from build123d import *

# Parameters (mm, degrees)
SKETCH_3_W          = 38
SKETCH_3_H          = 20
EXTRUDE_1_DEPTH     = 6
SKETCH_4_W          = 5
SKETCH_4_H          = 20
EXTRUDE_2_DEPTH     = 59
SKETCH_9_W          = 40.5
SKETCH_9_H          = 24.5
EXTRUDE_4_DEPTH     = 4
SKETCH_12_W         = 21.5
SKETCH_12_H         = 85
EXTRUDE_5_DEPTH     = 4
SKETCH_13_W         = 21.5
SKETCH_13_H         = 51
EXTRUDE_6_DEPTH     = 6
EXTRUDE_8_DEPTH     = 4
CUT_EXTRUDE_START   = -20
CUT_EXTRUDE_7_DEPTH = 8
SKETCH_5_R          = 2.1
CUT_EXTRUDE_1_DEPTH = 114.903467902
CUT_EXTRUDE_2_DEPTH = 3.8
SKETCH_7_R          = 2.6
CUT_EXTRUDE_3_DEPTH = 120.57529009
SKETCH_17_R         = 2.1
CUT_EXTRUDE_4_DEPTH = 165.903001792
CUT_EXTRUDE_5_DEPTH = 3.3
SKETCH_19_R         = 2.5
CUT_EXTRUDE_6_DEPTH = 118.123866056
FILLET_2_R          = 2.5
CHAMFER_2_SIZE      = 4


with BuildPart() as part:
    # Эскиз3 → Бобышка-Вытянуть1 (new body)
    with BuildSketch(Plane.XY):
        Rectangle(SKETCH_3_W, SKETCH_3_H)
    extrude(amount=EXTRUDE_1_DEPTH)

    # Эскиз4 → Бобышка-Вытянуть2 (add)
    with BuildSketch(Plane(origin=(-10.8, 0, 0), x_dir=(1, 0, 0), z_dir=(0, 0, 1))):
        with Locations((10.8, 0)):
            Rectangle(SKETCH_4_W, SKETCH_4_H)
    extrude(amount=-EXTRUDE_2_DEPTH)

    # Эскиз9 → Бобышка-Вытянуть4 (add)
    with BuildSketch(Plane.XY.offset(6)):
        with Locations((-17.75, 22.25)):
            Rectangle(SKETCH_9_W, SKETCH_9_H)
    extrude(amount=-EXTRUDE_4_DEPTH)

    # Эскиз12 → Бобышка-Вытянуть5 (add, symmetric)
    with BuildSketch(Plane(origin=(0, 10, 0), x_dir=(-1, 0, 0), z_dir=(0, 1, 0))):
        with Locations((8.25, 48.5)):
            Rectangle(SKETCH_12_W, SKETCH_12_H)
    extrude(amount=EXTRUDE_5_DEPTH, both=True)

    # Эскиз13 → Бобышка-Вытянуть6 (add)
    with BuildSketch(Plane.XY.offset(91)):
        with Locations((-8.25, 31.5)):
            Rectangle(SKETCH_13_W, SKETCH_13_H)
    extrude(amount=EXTRUDE_6_DEPTH)

    # Эскиз23 → Бобышка-Вытянуть8 (add)
    with BuildSketch(Plane(origin=(0, 10, 0), x_dir=(1, 0, 0), z_dir=(0, 1, 0))):
        Polygon((-2.5, 16.5), (-19, 0), (-2.5, 0), align=None)
    extrude(amount=-EXTRUDE_8_DEPTH)

    # Эскиз21 → Вырез-Вытянуть7 (cut)
    with BuildSketch(Plane(origin=(0, 0, -59), x_dir=(-1, 0, 0), z_dir=(0, 0, -1)).offset(CUT_EXTRUDE_START)):
        with BuildLine():
            Line((1.25, 10), (2.5, 10))
            Line((2.5, 10), (2.5, 8.75))
            ThreePointArc((2.5, 8.75), (2.133883476, 9.633883476), (1.25, 10))
        make_face()
    extrude(amount=-CUT_EXTRUDE_7_DEPTH, mode=Mode.SUBTRACT)

    # Эскиз5 → Вырез-Вытянуть1 (cut, through all)
    with BuildSketch(Plane.XY.offset(6)):
        with Locations((-9, -2)):
            Circle(SKETCH_5_R)
        with Locations((9, -2)):
            Circle(SKETCH_5_R)
    extrude(amount=-CUT_EXTRUDE_1_DEPTH, mode=Mode.SUBTRACT)

    # Эскиз6 → Вырез-Вытянуть2 (cut)
    with BuildSketch(Plane(origin=(0, 0, 0), x_dir=(-1, 0, 0), z_dir=(0, 0, -1))):
        Polygon((-9, 2.156921938), (-12.6, 0.078460969), (-12.6, -4.078460969), (-9, -6.156921938), (-5.4, -4.078460969), (-5.4, 0.078460969), align=None)
        Polygon((9, 2.156921938), (5.4, 0.078460969), (5.4, -4.078460969), (9, -6.156921938), (12.6, -4.078460969), (12.6, 0.078460969), align=None)
    extrude(amount=-CUT_EXTRUDE_2_DEPTH, mode=Mode.SUBTRACT)

    # Эскиз7 → Вырез-Вытянуть3 (cut, through all)
    with BuildSketch(Plane(origin=(2.5, 0, 0), x_dir=(0, 0, -1), z_dir=(1, 0, 0))):
        with Locations(Location((49, 0, 0), (0, 0, 90))):
            Circle(SKETCH_7_R)
    extrude(amount=-CUT_EXTRUDE_3_DEPTH, mode=Mode.SUBTRACT)

    # Эскиз17 → Вырез-Вытянуть4 (cut, through all)
    with BuildSketch(Plane(origin=(0, 0, 91), x_dir=(-1, 0, 0), z_dir=(0, 0, -1))):
        with Locations((7.5, 29)):
            Circle(SKETCH_17_R)
        with Locations((7.5, 47)):
            Circle(SKETCH_17_R)
    extrude(amount=-CUT_EXTRUDE_4_DEPTH, mode=Mode.SUBTRACT)

    # Эскиз18 → Вырез-Вытянуть5 (cut)
    with BuildSketch(Plane.XY.offset(97)):
        Polygon((-3.458548116, 29), (-5.479274058, 32.5), (-9.520725942, 32.5), (-11.541451884, 29), (-9.520725942, 25.5), (-5.479274058, 25.5), align=None)
        Polygon((-3.458548116, 47), (-5.479274058, 50.5), (-9.520725942, 50.5), (-11.541451884, 47), (-9.520725942, 43.5), (-5.479274058, 43.5), align=None)
    extrude(amount=-CUT_EXTRUDE_5_DEPTH, mode=Mode.SUBTRACT)

    # Эскиз19 → Вырез-Вытянуть6 (cut, through all)
    with BuildSketch(Plane(origin=(0, 0, 2), x_dir=(-1, 0, 0), z_dir=(0, 0, -1))):
        with Locations((30.999999999, 27.499999999)):
            Circle(SKETCH_19_R)
    extrude(amount=-CUT_EXTRUDE_6_DEPTH, mode=Mode.SUBTRACT)

    # Скругление2
    fillet_2_edges = [part.edges().sort_by_distance(p)[0] for p in [
        (0, 10, -59),
        (0, -10, -59),
        (2.5, 34.5, 4),
        (-38, 10, 4),
        (-38, 34.5, 4),
        (2.5, 57, 94),
        (-19, 57, 94),
        (19, 10, 3),
        (19, -10, 3),
        (-19, -10, 3),
    ]]
    fillet(fillet_2_edges, radius=FILLET_2_R)

    # Фаска2
    chamfer_2_edges = [part.edges().sort_by_distance(p)[0] for p in [
        (-19, 12, 6),
        (-8.25, 14, 91),
        (-8.25, 14, 6),
    ]]
    chamfer(chamfer_2_edges, length=CHAMFER_2_SIZE)


solid = part.part
Geometry: final body of the model. Coordinates: model frame, mm. A direction names the side the tool comes from. Coordinates: 2 decimals unless noted, no trailing zeros. Order: outer loops, then holes, each group sorted by start corner. A loop starts at its lowest first (then second) coordinate and runs counter-clockwise, first axis right, second up.
1) Section B-B (x = -31). Return loops of the section in (y, z).
Result sheet:
outline: (10, 2) - (25, 2) - (25, 6) - (10, 6) - close; (30, 2) - (34.5, 2) - (34.5, 6) - (30, 6) - close
2) Section D-D (z = 24.5). Return loops of the section in (x, y), then the cut area to 3 significant figures.
Result sheet:
outline: (-19, 6) - (2.5, 6) - (2.5, 14) - (-19, 14) - close
area: 172 mm2
3) Section C-C (x = -15). Return loops of the section in (y, z).
Result sheet:
outline: (-10, 0) - (6, 0) - (6, -4) - (10, -4) - (10, 2) - (34.5, 2) - (34.5, 6) - (18, 6) - (14, 10) - (14, 87) - (18, 91) - (57, 91) - (57, 97) - (6, 97) - (6, 6) - (-10, 6) - close
4) Set-up query: faces 1 (the flat face through (-7, 6, -5)), 2 (the flat face through (-8, 43.5, 95)), 3 (the flat face through (-8, 6, 51)), 4 (the flat face through (-18, 25, 6)). Return all of +Z, -Z, +X, -X, +Y, -Y with unobstructed straight access to the full face (end or side cutting, diameter ignored); none if empty.
Result sheet:
face 1: -Z, -X, -Y
face 2: +Z
face 3: +Z, +X, -X, -Y
face 4: -X, +Y
5) Section A-A (z = -49). Return loops of the section in (x, y).
Result sheet:
outline: (-2.5, -10) - (2.5, -10) - (2.5, -2.6) - (-2.5, -2.6) - close; (-2.5, 2.6) - (2.5, 2.6) - (2.5, 10) - (-2.5, 10) - close
6) Ray query, probe 1 along Y at (x, z) = (-7.5, 91.65); probe 2 along Y at (x, z) = (-9, 4); probe 3 along X at (y, z) = (-2, -13). Return the intervals inside material, ascending.
Result sheet:
probe 1: y = 6 to 26.9, 31.1 to 44.9, 49.1 to 57
probe 2: y = -10 to -4.1, 0.1 to 34.5
probe 3: x = -2.5 to 2.5
7) Draft query along Y for faces 5 (the flat face through (-7, -5, 2)), 6 (the flat face through (0, 0, -59)), 7 (the flat face through (-18, 34.5, 4)). Return one class per face: released by +Y, released by -Y, zero draft, split by the parting line, or undercut.
Result sheet:
face 5: undercut
face 6: zero draft
face 7: released by +Y
8) First-contact query: P1, Ø3.5, axis at x = -8.5, y = -3.5, coming from the -Z side; P2, Ø10, axis at y = -4, z = -38.5, coming from the -X side; P3, Ø5, axis at x = -4.5, y = 25.5, coming from the -Z side. Flat tips, straight axial feed; report the tip coordinate or a pass-through.
Result sheet:
P1: stops at z = 3.8
P2: stops at x = -2.5
P3: stops at z = 2
